Part model, mm, in its own coordinate system. Coordinates: 2 decimals unless noted, no trailing zeros. Loops run counter-clockwise (first coordinate to the right, second up) from the corner with the lowest first, then second, coordinate; pieces in that order, holes last. Notation, with made-up numbers: (-33.5, -12.5) - (19.5, -12.5) arc R12 cw to (19.5, 7.5) - close; hole circle Ø6 at (9.25, 82). An arc over 180 degrees is marked (long way). Use a Markdown table: item, result. Add a question column.
1) Band-saw the part on A-A (x = -882.5). Give the cut face in (y, z), plus the area to 3 significant figures.
2) Band-saw the part on B-B (y = -51). Give the cut face in (x, z), plus the area to 3 significant figures.
3) Drop flat-ended pins along their axis: P1, Ø10, axis at x = -647, y = 53, coming from the -Z side; P2, Ø10, axis at y = 28.5, z = 19.5, coming from the +X side; P3, Ø10, axis at x = -120.65, y = 0, coming from the -Z side. Give the stop position or say it passes through.
4) Probe probe 1 along Y at (x, z) = (-120, 12); probe 2 along Z at (x, y) = (-626.5, 82); probe 3 along X at (y, z) = (-104, 29). List the from-to ranges inside material, lowest first. Write a range as [from, to].
from build123d import *

# Parameters (mm, degrees)
F0_R     = 6.35
F1_DEPTH = 31.75
F2_R     = 6.35
F3_DEPTH = 6.35
F5_DEPTH = 31.75


with BuildPart() as f1:
    # F0 (on Top) → F1 (new body)
    with BuildSketch(Plane.XY):
        with BuildLine():
            Line((-1136.65, 120.65), (-1136.65, -120.65))
            Line((-1136.65, -120.65), (-120.65, -120.65))
            ThreePointArc((-120.65, -120.65), (0, 0), (-120.65, 120.65))
            Line((-120.65, 120.65), (-1136.65, 120.65))
        make_face()
        with Locations((-120.65, 0)):
            Circle(F0_R, mode=Mode.SUBTRACT)
    extrude(amount=F1_DEPTH)

    # F2 (on face) → F3 (join)
    with BuildSketch(Plane(origin=(0, 0, 0), x_dir=(1, 0, 0), z_dir=(0, 0, -1))):
        with Locations((-400.05, 114.3)):
            Circle(F2_R)
    extrude(amount=F3_DEPTH)

    # F4 (on face) → F5 (cut)
    with BuildSketch(Plane(origin=(0, 0, 0), x_dir=(1, 0, 0), z_dir=(0, 0, -1))):
        with BuildLine():
            Line((-393.446, -120.65), (-393.446, -114.046))
            ThreePointArc((-393.446, -114.046), (-400.05, -107.442), (-406.654, -114.046))
            Line((-406.654, -114.046), (-406.654, -120.65))
            Line((-406.654, -120.65), (-393.446, -120.65))
        make_face()
    extrude(amount=-F5_DEPTH, mode=Mode.SUBTRACT)


solid = f1.part
Answer block:
| question | item | result |
|---|---|---|
| 1 | outline | (-120.65, 0) - (120.65, 0) - (120.65, 31.75) - (-120.65, 31.75) - close |
| 1 | area | 7,660 mm2 |
| 2 | outline | (-1136.65, 0) - (-11.31, 0) - (-11.31, 31.75) - (-1136.65, 31.75) - close |
| 2 | area | 35,700 mm2 |
| 3 | P1 | z = 0 |
| 3 | P2 | x = -2.31 |
| 3 | P3 | through |
| 4 | probe 1 | [-120.65, -6.32], [6.32, 120.65] |
| 4 | probe 2 | [0, 31.75] |
| 4 | probe 3 | [-1136.65, -59.49] |
